```python
from build123d import *

# Parameters (mm, degrees)
F1_DEPTH = 75
F2_F1_R  = 5
F2_F2_R  = 5
F2_F3_R  = 5
F2_F4_R  = 5


# Not quite as in the source:
# - a feature of the source that left no trace in its solid (it failed there, or was rolled back) is left out


with BuildPart() as f1:
    # F0 (on Right) → F1 (new body, symmetric)
    with BuildSketch(Plane.YZ):
        Polygon((-15.2537021786, 50), (17.912545725, 0), (37.912545725, 0), (4.7462978214, 50), align=None)
    extrude(amount=F1_DEPTH, both=True)

    # F2: fillet of radius 5 on 4 edges, made by hand

    # F2_f1
    f2_f1_edges = [f1.edges().sort_by_distance(p)[0] for p in [
        (0, -15.2537021786, 50),
    ]]
    fillet(f2_f1_edges, radius=F2_F1_R)

    # F2_f2
    f2_f2_edges = [f1.edges().sort_by_distance(p)[0] for p in [
        (0, 4.7462978214, 50),
    ]]
    fillet(f2_f2_edges, radius=F2_F2_R)

    # F2_f3
    f2_f3_edges = [f1.edges().sort_by_distance(p)[0] for p in [
        (-75, -1.9370773882, 50),
    ]]
    fillet(f2_f3_edges, radius=F2_F3_R)

    # F2_f4
    f2_f4_edges = [f1.edges().sort_by_distance(p)[0] for p in [
        (75, -1.9370773882, 50),
    ]]
    fillet(f2_f4_edges, radius=F2_F4_R)


solid = f1.part
```
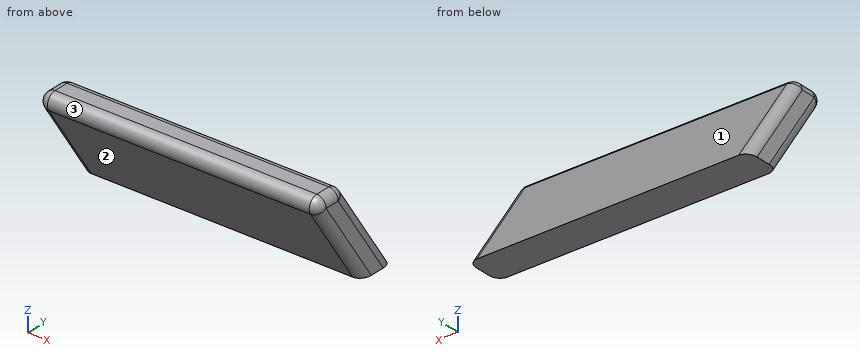
Geometry check sheet. Reference: the model listing, model coordinates, mm. Face numbers are marked on the shaded views. Coordinates: 2 decimals unless noted, no trailing zeros. Order: outer loops, then holes, each group sorted by start corner. A loop starts at its lowest first (then second) coordinate and runs counter-clockwise, first axis right, second up.
Item 1: Section check A-A (x = 28). Enter the section's corners in (y, z).
Item 2: Mould release check, pull along Z, two halves, no side actions. Record for the marked faces 1, 2 and 3: released by +Z, released by -Z, zero draft, split by the parting line, or undercut.
Item 3: Depth check by flat-ended pin: pin 1 (6 mm diameter, centred on x = 44.5, z = 30.5, fed in from -Y); pin 2 (5 mm diameter, centred on x = -57.5, y = 0.5, fed in from -Z); pin 3 (4 mm diameter, centred on x = 50.5, z = 24.5, fed in from +Y). Enter the tip coordinate at first touch or a pass-through.
Item 4: Scan lines: line 1 along Y through (x, z) = (-43, 32.5); line 2 along Z through (x, y) = (-53.5, 25.5); line 3 along Z through (x, y) = (57, 5.5). Record each from-to range of solid material in increasing order.
Check sheet entries:
1. outline: (-10.1, 42.24) - (17.91, 0) - (37.91, 0) - (6.23, 47.76) arc R5 ccw to (2.06, 50) - (-5.94, 50) arc R5 ccw to start
2. face 1: released by +Z
2. face 2: released by -Z
2. face 3: split by the parting line
3. pin 1: stops at y = -4.31
3. pin 2: stops at z = 22.48
3. pin 3: stops at y = 22.99
4. line 1: y = -3.65 to 16.35
4. line 2: z = 0 to 18.71
4. line 3: z = 18.71 to 48.63
